Job drawing, mm, ordinate dimensions from the low corner. One solid piece. A direction names the side the tool comes from. Round coordinates to 2 decimals unless told otherwise and drop trailing zeros. Loops run counter-clockwise (first coordinate to the right, second up) from the corner with the lowest first, then second, coordinate; pieces in that order, holes last.
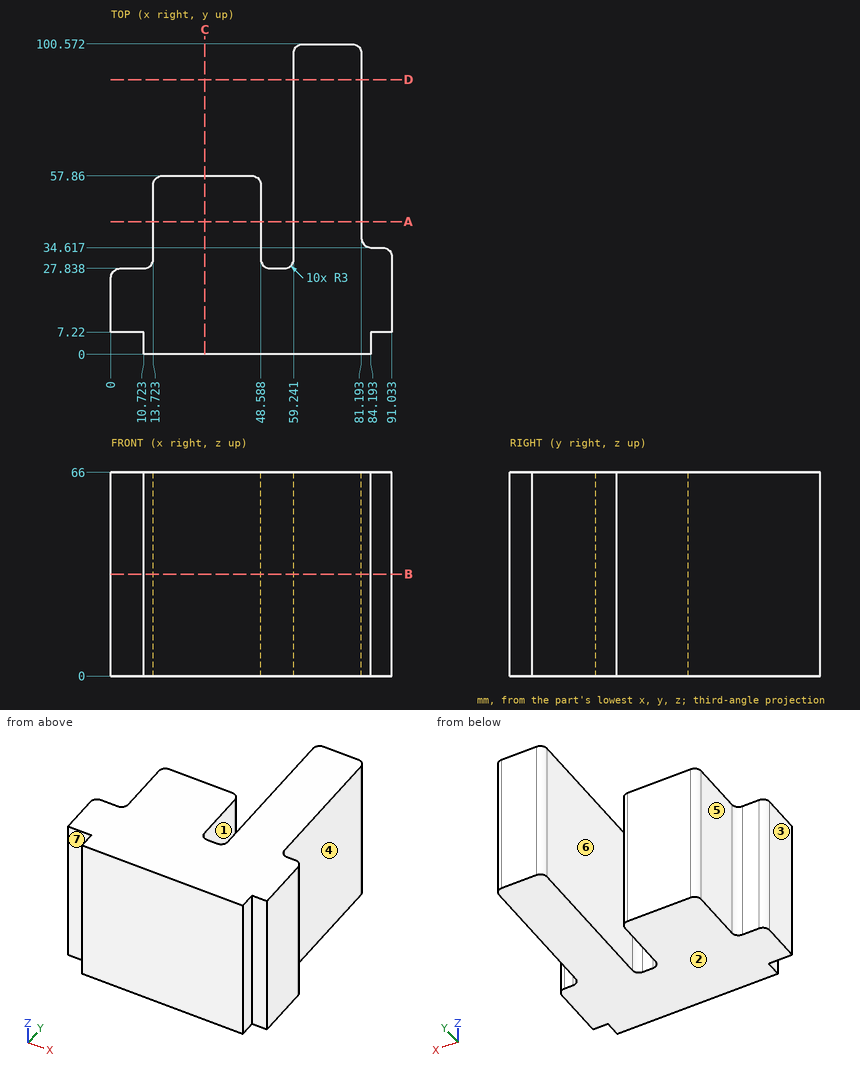
Item 1: Two-plate mould, pull along X, no slides. Class the marked faces 1, 2, 3 and 4: released by +X, released by -X, zero draft, split by the parting line, or undercut.
Answers follow:
face 1: undercut
face 2: zero draft
face 3: released by -X
face 4: released by +X
Item 2: Cut at D-D, the plane y = 89. Give the cut face in (x, z).
Answers follow:
outline: (59.24, 0) - (81.19, 0) - (81.19, 66) - (59.24, 66) - close
Item 3: Flat gauge pins, fed straight in: P1, Ø3, axis at x = 86, z = 19.5, coming from the +Y side; P2, Ø6, axis at y = 2, z = 42, coming from the -X side; P3, Ø6, axis at y = 2, z = 48, coming from the +X side; P4, Ø2, axis at x = 35, y = 52.5, coming from the -Z side. Where does each tip first touch, or does it go through?
Answers follow:
P1: stops at y = 34.62
P2: stops at x = 10.72
P3: stops at x = 84.19
P4: stops at z = 0
Item 4: 3-axis set-ups, long thin cutter, end or side, ignore diameter. For the marked faces 5, 6 and 7: which of +Z, -Z, +X, -X, +Y, -Y reach the whole face in a straight line?
Answers follow:
face 5: +Z, -Z, -X, +Y
face 6: +Z, -Z, +Y
face 7: +Z, -Z, -X, -Y
Item 5: Cut at C-C, the plane x = 30.5. Give the cut face in (y, z).
Answers follow:
outline: (0, 0) - (57.86, 0) - (57.86, 66) - (0, 66) - close
Item 6: Cut at B-B, the plane z = 33. Give the cut face in (x, y).
Answers follow:
outline: (0, 7.22) - (10.72, 7.22) - (10.72, 0) - (84.19, 0) - (84.19, 7.22) - (91.03, 7.22) - (91.03, 31.62) arc R3 ccw to (88.03, 34.62) - (84.19, 34.62) arc R3 cw to (81.19, 37.62) - (81.19, 97.57) arc R3 ccw to (78.19, 100.57) - (62.24, 100.57) arc R3 ccw to (59.24, 97.57) - (59.24, 30.84) arc R3 cw to (56.24, 27.84) - (51.59, 27.84) arc R3 cw to (48.59, 30.84) - (48.59, 54.86) arc R3 ccw to (45.59, 57.86) - (16.72, 57.86) arc R3 ccw to (13.72, 54.86) - (13.72, 30.84) arc R3 cw to (10.72, 27.84) - (3, 27.84) arc R3 ccw to (0, 24.84) - close
Item 7: Probe line 1 (X direction, y = 50, z = 63); line 2 (X direction, y = 65, z = 41); line 3 (Y direction, x = 43, z = 50.5). List the from-to ranges inside material, lowest first.
Answers follow:
line 1: x = 13.72 to 48.59, 59.24 to 81.19
line 2: x = 59.24 to 81.19
line 3: y = 0 to 57.86
Item 8: Cut at A-A, the plane y = 43. Give the cut face in (x, z), plus the area to 3 significant figures.
Answers follow:
outline: (13.72, 0) - (48.59, 0) - (48.59, 66) - (13.72, 66) - close; (59.24, 0) - (81.19, 0) - (81.19, 66) - (59.24, 66) - close
area: 3,750 mm2
